Could you check a few things on this model? Use its own coordinates, in mm. Face numbers are marked on the shaded views. A direction names the side the tool comes from. Coordinates: 2 decimals unless noted, no trailing zeros. Write each loop counter-clockwise with the first axis right and the second up, starting at its lowest first coordinate (ties: lowest second). Pieces come first, ordered by that corner, then holes. Notation, with made-up numbers: M 67.5,-1.75 L 121.5,-1.75 A22 ccw 121.5,6.25 Z; hole C 86.25,35 d2. An arc over 180 degrees is marked long. Write item = value, one per line.
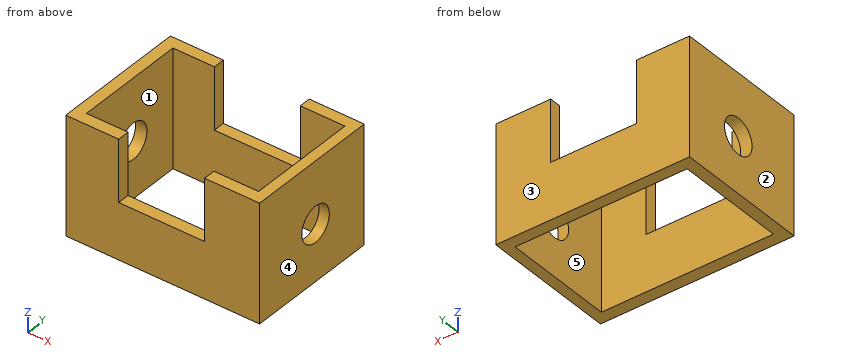
```python
from build123d import *

# Parameters (mm, degrees)
F0_W     = 182.2371855378
F0_H     = 110.8047105372
F1_DEPTH = 127
F2_W     = 80.7708539069
F2_H     = 63.6986494064
F3_DEPTH = 127.001
F4_W     = 161.728402134
F4_H     = 104.781774804
F5_DEPTH = 110.8057105372
F6_R     = 16.7086573523
F7_DEPTH = 182.2381855378


with BuildPart() as f1:
    # F0 (on Front) → F1 (new body)
    with BuildSketch(Plane.XZ):
        with Locations((4.7809146345, 2.6716869324)):
            Rectangle(F0_W, F0_H)
    extrude(amount=-F1_DEPTH)

    # F2 (on Front) → F3 (cut, through all)
    with BuildSketch(Plane.XZ):
        with Locations((3.8164127618, 31.8493247032)):
            Rectangle(F2_W, F2_H)
    extrude(amount=-F3_DEPTH, mode=Mode.SUBTRACT)

    # F4 (on face) → F5 (cut, through all)
    with BuildSketch(Plane(origin=(0, 0, -52.7306683362), x_dir=(1, 0, 0), z_dir=(0, 0, -1))):
        with Locations((5.3121293895, -63.7166202068)):
            Rectangle(F4_W, F4_H)
    extrude(amount=-F5_DEPTH, mode=Mode.SUBTRACT)

    # F6 (on face) → F7 (cut, through all)
    with BuildSketch(Plane.YZ.offset(95.8995074034)):
        with Locations((67.9201483727, 0)):
            Circle(F6_R)
    extrude(amount=-F7_DEPTH, mode=Mode.SUBTRACT)


solid = f1.part
```
Item 1: I'm going to push a flat-ended pin straight in: P1, Ø9, axis at x = -6.5, y = 3.5, coming from the +Z side. Where does the tip first touch, or does it pass through?
Numbers:
P1 = 0
Item 2: For the marked faces 4 and 5, which set-ups out of +Z, -Z, +X, -X, +Y, -Y let a thin tool reach every point of the face, with its end or its side?
Numbers:
face_4 = +Z, -Z, +X, +Y, -Y
face_5 = +Z, -Z
Item 3: Imagine slicing it at D-D (z = -25). Write out the boundary of the cut face in (x, y).
Numbers:
outline = M -86.34,0 L 95.9,0 L 95.9,127 L -86.34,127 Z; hole M -75.55,11.33 L 86.18,11.33 L 86.18,116.11 L -75.55,116.11 Z
Item 4: If I drill on line 1 along Y through (x, z) = (60.5, 24); line 2 along X through (y, z) = (43, 18.5); line 3 along X through (y, z) = (6.5, 7.5), over which ranges is the centre line in solid material (lowest first)?
Numbers:
line_1 = 0 to 11.33, 116.11 to 127
line_2 = -86.34 to -75.55, 86.18 to 95.9
line_3 = -86.34 to -36.57, 44.2 to 95.9
Item 5: If we mould it in two halves opening along X, with no side actions, what happens to the marked faces 1, 2 and 3? For each: pulls with the +X half, pulls with the -X half, needs draft (parallel to the pull), parting line crosses it, or undercut.
Numbers:
face_1 = undercut
face_2 = pulls with the -X half
face_3 = needs draft
Item 6: Imagine slicing it at B-B (x = -65). Write out the boundary of the cut face in (y, z), and give its area (3 significant figures).
Numbers:
outline = M 0,-52.73 L 11.33,-52.73 L 11.33,58.07 L 0,58.07 Z; M 116.11,-52.73 L 127,-52.73 L 127,58.07 L 116.11,58.07 Z
area = 2,460 mm²
Item 7: Imagine slicing it at A-A (z = 47.5). Write out the boundary of the cut face in (x, y).
Numbers:
outline = M -86.34,0 L -36.57,0 L -36.57,11.33 L -75.55,11.33 L -75.55,116.11 L -36.57,116.11 L -36.57,127 L -86.34,127 Z; M 44.2,0 L 95.9,0 L 95.9,127 L 44.2,127 L 44.2,116.11 L 86.18,116.11 L 86.18,11.33 L 44.2,11.33 Z
Item 8: Imagine slicing it at C-C (y = 14). Write out the boundary of the cut face in (x, z).
Numbers:
outline = M -86.34,-52.73 L -75.55,-52.73 L -75.55,58.07 L -86.34,58.07 Z; M 86.18,-52.73 L 95.9,-52.73 L 95.9,58.07 L 86.18,58.07 Z
